Could you check a few things on this model? Use its own coordinates, in mm. A direction names the side the tool comes from. Give positions to 0.01 mm unless a question says otherwise; leave off trailing zeros. Loops run counter-clockwise (first coordinate to the right, second up) from the corner with the lowest first, then second, coordinate; pieces in that order, holes last. Notation, with made-up numbers: (12.5, 67.5) -> (64.5, 67.5) arc R22 ccw to (64.5, 84.5) -> close; hole circle Ø5 at (31.5, -19). An arc over 180 degrees is marked (long way). Put each result on its own line as item: value.
Autodesk Inventor part; units mm, degrees
ref_plane "YZ Plane" through (0, 0, 0) normal (1, 0, 0) x (0, 1, 0)
ref_plane "XZ Plane" through (0, 0, 0) normal (0, 1, 0) x (-1, 0, 0)
ref_plane "XY Plane" through (0, 0, 0) normal (0, 0, 1) x (1, 0, 0)
sketch "Szkic1" plane through (0, 0, 0) normal (0, 0, 1) x (1, 0, 0)
  circle A0 centre (0, 0) radius 24
  dimension "d0" = 48
extrude "Wyciągnięcie proste1" add sketch "Szkic1" along normal blind 10
sketch "Szkic2" plane through (0, 0, 10) normal (0, 0, 1) x (1, 0, 0)
  circle A0 centre (0, 0) radius 14
  dimension "d3" = 28
extrude "Wyciągnięcie proste2" add sketch "Szkic2" along normal blind 50
sketch "Szkic3" plane through (0, 0, 60) normal (0, 0, 1) x (1, 0, 0)
  circle A0 centre (0, 0) radius 8
  dimension "d6" = 16
extrude "Wyciągnięcie proste3" cut sketch "Szkic3" against normal through all
sketch "Szkic4" plane through (0, 0, 10) normal (0, 0, 1) x (1, 0, 0)
  line L0 (-34.1509, 26.2264) -> (-20, 26.2264)
  line L1 (-20, 26.2264) -> (-20, -20.7547)
  line L2 (-20, -20.7547) -> (-34.1509, -20.7547)
  line L3 (-34.1509, -20.7547) -> (-34.1509, 26.2264)
  line L4 (20, 30.566) -> (32.0755, 30.566)
  line L5 (32.0755, 30.566) -> (32.0755, -32.8302)
  line L6 (32.0755, -32.8302) -> (20, -32.8302)
  line L7 (20, -32.8302) -> (20, 30.566)
  point P0 (0, 0)
  dimension "d9" = 40
  dimension "d10" = 20
extrude "Wyciągnięcie proste4" cut sketch "Szkic4" against normal blind 40
sketch "Szkic5" plane through (0, 0, 10) normal (0, 0, 1) x (1, 0, 0)
  circle A0 centre (0, 0) radius 19
  circle A1 centre (0, 19) radius 2.75
  circle A2 centre (13.435, 13.435) radius 2.75
  circle A3 centre (-13.435, 13.435) radius 2.75
  line L0 (0, 0) -> (-30.3885, 30.3885)
  line L1 (0, 0) -> (37.6377, 37.6377)
  line L2 (0, 0) -> (34.9843, 0)
  dimension "d13" = 38
  dimension "d14" = 5.5
  dimension "d15" = 5.5
  dimension "d16" = 5.5
  dimension "d17" = 45
  dimension "d18" = 90
extrude "Wyciągnięcie proste5" cut sketch "Szkic5" against normal blind 40 contours A2 L1 A0 | A0 L1 A2 | A3 L0 A0 | A0 L0 A3 | L1 A2 A0 | A0 A2 L1 | L0 A3 A0 | A0 A3 L0 | A1 A0 | A0 A1
mirror "Odbij1" about plane through (0, 0, 0) normal (0, 1, 0) of "Wyciągnięcie proste5"
properties part number "Cartesian1_BallNut" material "Stal, stopowa"
1. If we section it at C-C (x = -12): List the corners of the cut face in (y, z) for me, then the cut area to 3 significant figures.
Recorded:
outline: (-20.78, 0) -> (-15.78, 0) -> (-15.78, 10) -> (-20.78, 10) -> close; (-11.09, 0) -> (11.09, 0) -> (11.09, 10) -> (7.21, 10) -> (7.21, 60) -> (-7.21, 60) -> (-7.21, 10) -> (-11.09, 10) -> close; (15.78, 0) -> (20.78, 0) -> (20.78, 10) -> (15.78, 10) -> close
area: 1,040 mm^2
2. If we section it at D-D (z = 28): List the corners of the cut face in (x, y) for me.
Recorded:
outline: circle Ø28 at (0, 0); hole circle Ø16 at (0, 0)
3. Thinking about a two-plate mould opening in X: for faces 3 (the face through (9, 0, 0)), 4 (the face through (20, 0, 5)), 5 (the face through (-1.73, -7.81, 30.42)), which applies, pulls with the +X half, pulls with the -X half, needs draft (parallel to the pull), parting line crosses it, or undercut?
Recorded:
face 3: needs draft
face 4: pulls with the +X half
face 5: undercut
4. I'm going to push flat-ended pins straight in: pin 1 (1 mm diameter, centred on x = -11, y = 13, fed in from +Z); pin 2 (4 mm diameter, centred on x = -3.5, z = 14.5, fed in from +Y); pin 3 (2 mm diameter, centred on y = -15.5, z = 8.5, fed in from -X). Where does each tip first touch, or does it pass through?
Recorded:
pin 1: stops at z = 10
pin 2: stops at y = 13.92
pin 3: stops at x = -19.12
5. If we section it at A-A (x = 0): List the corners of the cut face in (y, z) for me, then the cut area to 3 significant figures.
Recorded:
outline: (-24, 0) -> (-21.75, 0) -> (-21.75, 10) -> (-24, 10) -> close; (-16.25, 0) -> (-8, 0) -> (-8, 60) -> (-14, 60) -> (-14, 10) -> (-16.25, 10) -> close; (8, 0) -> (16.25, 0) -> (16.25, 10) -> (14, 10) -> (14, 60) -> (8, 60) -> close; (21.75, 0) -> (24, 0) -> (24, 10) -> (21.75, 10) -> close
area: 810 mm^2
6. For faces 1 (the face through (-9, 11, 10)), 2 (the face through (11.408, 15.294, 5.07)), which set-ups out of +Z, -Z, +X, -X, +Y, -Y let a thin tool reach every point of the face, with its end or its side?
Recorded:
face 1: +Z
face 2: +Z, -Z
7. If we section it at B-B (y = 0): List the corners of the cut face in (x, z) for me.
Recorded:
outline: (-20, 0) -> (-8, 0) -> (-8, 60) -> (-14, 60) -> (-14, 10) -> (-20, 10) -> close; (8, 0) -> (20, 0) -> (20, 10) -> (14, 10) -> (14, 60) -> (8, 60) -> close
8. I need wall thicknesses on line 1 (Y direction, x = 0, z = 19); line 2 (Z direction, x = -5, y = -21); line 3 (Y direction, x = 15.5, z = 9.5). Which ranges of each line are inside material? Lowest first, please.
Recorded:
line 1: y = -14 to -8, 8 to 14
line 2: z = 0 to 10
line 3: y = -18.32 to -15.25, -11.62 to 11.62, 15.25 to 18.32
